Design review of the part built by this model. Coordinates are the model's own, in mm. A direction names the side the tool comes from. Give positions to 0.01 mm unless a question says otherwise; leave off trailing zeros. Order: outer loops, then holes, each group sorted by start corner. A loop starts at its lowest first (then second) coordinate and runs counter-clockwise, first axis right, second up. Notation, with made-up numbers: M 42.5,52 L 83.5,52 A26 cw 83.5,86 Z; hole C 82,67.5 d9. An arc over 180 degrees is marked long. Answer as a JSON object with one key per item and string values.
from build123d import *

# Parameters (mm, degrees)
F0_W     = 140.7188475132
F0_H     = 52.7415163815
F1_DEPTH = 25.4
F2_R     = 8.9116900181
F3_DEPTH = 25.4
F4_T     = -2.54


with BuildPart() as f1:
    # F0 (on Top) → F1 (new body)
    with BuildSketch(Plane.XY):
        with Locations((1.1782646179, 2.4687517434)):
            Rectangle(F0_W, F0_H)
    extrude(amount=F1_DEPTH)

    # F2 (on face) → F3 (join)
    with BuildSketch(Plane.XY.offset(25.4)):
        with Locations((43.2196445763, -4.8853275366)):
            Circle(F2_R)
    extrude(amount=F3_DEPTH)

    # F4
    f4_openings = [f1.faces().sort_by_distance(p)[0] for p in [
        (71.537688, 2.468752, 12.7),
    ]]
    offset(amount=F4_T, openings=f4_openings, kind=Kind.INTERSECTION)


solid = f1.part
(1) We need section C-C (y = -17). Write out the cut boundary in (x, z), plus the area to 3 significant figures.
Checked values:
{"outline": "M -69.18,0 L 71.54,0 L 71.54,2.54 L -66.64,2.54 L -66.64,22.86 L 71.54,22.86 L 71.54,25.4 L -69.18,25.4 Z", "area": "766 mm^2"}
(2) We need section B-B (z = 4). Write out the cut boundary in (x, y), plus the area to 3 significant figures.
Checked values:
{"outline": "M -69.18,-23.9 L 71.54,-23.9 L 71.54,-21.36 L -66.64,-21.36 L -66.64,26.3 L 71.54,26.3 L 71.54,28.84 L -69.18,28.84 Z", "area": "836 mm^2"}
(3) Draft analysis for pull direction Y (two halves, no side actions). For faces 4 (the flat face through (0, 3, 25.4)), 5 (the cylindrical face through (51.45, -8.3, 37.92)), 6 (the flat face through (1, 3, 2.54)), state which applies: +Y half, -Y half, draft (parallel to the pull), parting line (faces both ways), or undercut.
Checked values:
{"face 4": "draft", "face 5": "parting line", "face 6": "undercut"}
(4) We need section A-A (x = 15). Write out the cut boundary in (y, z).
Checked values:
{"outline": "M -23.9,0 L 28.84,0 L 28.84,25.4 L -23.9,25.4 Z; hole M -21.36,2.54 L 26.3,2.54 L 26.3,22.86 L -21.36,22.86 Z"}
(5) To check wall thickness, follow L1, parallel to Y at x = -46.5, z = 3.5; L2, parallel to Z at x = 7.5, y = 12.5; L3, parallel to X at y = -8, z = 47. State the ranges of each line that lie inside material, in increasing order. Write a range as from..to.
Checked values:
{"L1": "y = -23.9..-21.36, 26.3..28.84", "L2": "z = 0..2.54, 22.86..25.4", "L3": "x = 34.87..37.66, 48.78..51.57"}
(6) We need section D-D (z = 36.5). Write out the cut boundary in (x, y).
Checked values:
{"outline": "C 43.22,-4.89 d17.82; hole C 43.22,-4.89 d12.74"}
(7) Tool access review of faces 1 (the flat face through (1, 3, 22.86)), 2 (the flat face through (43, -5, 50.8)), 3 (the flat face through (43, -5, 48.26)): name each direction out of +Z, -Z, +X, -X, +Y, -Y from which nothing blocks a thin tool from reaching the whole face with its end or side.
Checked values:
{"face 1": "+X", "face 2": "+Z, +X, -X, +Y, -Y", "face 3": "none"}
(8) Insertion check: pin 1 (3 mm diameter, centred on y = -8.5, z = 28.5, fed in from -X); pin 2 (2 mm diameter, centred on x = 30, y = -1.5, fed in from +Z). Each pin has a flat end and moves straight along its axis. Give the tip position at first contact, or say it passes through.
Checked values:
{"pin 1": "stops at x = 34.56", "pin 2": "stops at z = 25.4"}
